Autodesk Inventor part; units mm, degrees
ref_plane "YZ Plane" through (0, 0, 0) normal (1, 0, 0) x (0, 1, 0)
ref_plane "XZ Plane" through (0, 0, 0) normal (0, 1, 0) x (-1, 0, 0)
ref_plane "XY Plane" through (0, 0, 0) normal (0, 0, 1) x (1, 0, 0)
sketch "Sketch1" plane through (0, 0, 0) normal (0, 0, 1) x (1, 0, 0)
  circle A0 centre (0, 0) radius 3.5 construction
  circle A1 centre (0, 0) radius 4.5 construction
  line L0 (0, 0) -> (4.5, 0) construction
  line L1 (4.5, 0) -> (4.5, 3.5) construction
  line L2 (4.5, 3.5) -> (0, 3.5) construction
  line L3 (0, 3.5) -> (0, 0) construction
  line L4 (4.5, 3.5) -> (-4.5, 3.5)
  line L5 (-4.5, 3.5) -> (-4.5, -3.5)
  line L6 (-4.5, -3.5) -> (4.5, -3.5)
  line L7 (4.5, -3.5) -> (4.5, 3.5)
  line L8 (-4.5, 3.5) -> (-6, 3.5) construction
  line L9 (-6, 3.5) -> (-6, -3.5) construction
  line L10 (-6, -3.5) -> (-4.5, -3.5) construction
  line L11 (-4.5, -3.5) -> (-4.5, 3.5) construction
  line L12 (-6, 3.5) -> (4.5, 3.5) construction
  line L13 (4.5, 3.5) -> (4.5, 4.3) construction
  line L14 (4.5, 4.3) -> (-6, 4.3) construction
  line L15 (-6, 4.3) -> (-6, 3.5) construction
  line L16 (-6, -3.5) -> (4.5, -3.5) construction
  line L17 (4.5, -3.5) -> (4.5, -4.3) construction
  line L18 (4.5, -4.3) -> (-6, -4.3) construction
  line L19 (-6, -4.3) -> (-6, -3.5) construction
  line L20 (4.5, -4.3) -> (5.3, -4.3) construction
  line L21 (5.3, -4.3) -> (5.3, 4.3) construction
  line L22 (5.3, 4.3) -> (4.5, 4.3) construction
  line L23 (4.5, 4.3) -> (4.5, -4.3) construction
  line L24 (-6, 4.3) -> (5.3, 4.3)
  line L25 (5.3, 4.3) -> (5.3, -4.3)
  line L26 (5.3, -4.3) -> (-6, -4.3)
  line L27 (-6, -4.3) -> (-6, 4.3)
  dimension "d0" = 7
  dimension "d1" = 9
  dimension "d2" = 4.5
  dimension "d3" = 3.5
  dimension "d4" = 1.5
  dimension "d5" = 0.8
  dimension "d6" = 0.8
  dimension "d7" = 0.8
extrude "Extrusion1" add sketch "Sketch1" along normal blind 3.5
sketch "Sketch2" plane through (0, 0, 3.5) normal (0, 0, 1) x (1, 0, 0)
  line L0 (5.3, -4.3) -> (-6, -4.3)
  line L1 (-6, 4.3) -> (-4.5, 4.3)
  line L2 (-4.5, 4.3) -> (-4.5, -4.3)
  line L3 (-4.5, -4.3) -> (-6, -4.3)
  line L4 (-6, -4.3) -> (-6, 4.3)
  point P0 (0, 0)
extrude "Extrusion2" cut sketch "Sketch2" against normal blind 2.25
sketch "Sketch3" plane through (0, 0, 3.5) normal (0, 0, 1) x (1, 0, 0)
  line L0 (-4.5, -3.5) -> (-4.5, -4.3)
  line L1 (5.3, -4.3) -> (-4.5, -4.3)
  line L2 (5.3, 4.3) -> (5.3, -4.3)
  line L3 (-4.5, 4.3) -> (5.3, 4.3) construction
  line L4 (5.3, 4.3) -> (5.3, 3.9) construction
  line L5 (5.3, 3.9) -> (-4.5, 3.9) construction
  line L6 (-4.5, 3.9) -> (-4.5, 4.3) construction
  line L7 (5.3, 4.3) -> (4.9, 4.3) construction
  line L8 (4.9, 4.3) -> (4.9, -4.3) construction
  line L9 (4.9, -4.3) -> (5.3, -4.3) construction
  line L10 (5.3, -4.3) -> (5.3, 4.3) construction
  line L11 (5.3, -4.3) -> (-4.5, -4.3) construction
  line L12 (-4.5, -4.3) -> (-4.5, -3.9) construction
  line L13 (-4.5, -3.9) -> (5.3, -3.9) construction
  line L14 (5.3, -3.9) -> (5.3, -4.3) construction
  line L15 (-4.5, 3.9) -> (-4.5, 4.3)
  line L16 (5.3, 4.3) -> (5.3, -4.3)
  line L17 (-4.5, -4.3) -> (-4.5, -3.9)
  line L18 (4.9, -3.9) -> (4.9, 3.9)
  line L19 (4.9, 3.9) -> (-4.5, 3.9)
  line L20 (-4.5, 4.3) -> (5.3, 4.3)
  line L21 (4.9, -3.9) -> (-4.5, -3.9)
  line L22 (-4.5, -4.3) -> (5.3, -4.3)
  point P0 (0, 0)
  dimension "d12" = 0.4
  dimension "d13" = 0.4
  dimension "d14" = 0.4
extrude "Extrusion3" cut sketch "Sketch3" against normal blind 0.8
sketch "Sketch4" plane through (-6, -4.3, 0) normal (0, -1, 0) x (1, 0, 0)
  line L0 (11.3, 2.7) -> (1.5, 2.7)
  line L1 (11.3, 0) -> (0, 0)
  line L2 (12.285, 1.4959) -> (-1.3636, 1.4959) construction
  line L3 (6, 1.4959) -> (8, 1.4959) construction
  line L4 (8, 2.7) -> (6, 2.7) construction
  line L5 (8, 2.7) -> (4, 2.7)
  line L6 (1.5, 2.7) -> (2.5, 2.7) construction
  line L7 (2.5, 2.7) -> (2.5, 0) construction
  line L8 (2.5, 0) -> (1.5, 0) construction
  line L9 (1.5, 0) -> (1.5, 2.7) construction
  line L10 (2.5, 2.7) -> (6.5, 2.7)
  line L11 (6.5, 2.7) -> (6.5, 0)
  line L12 (6.5, 0) -> (2.5, 0)
  line L13 (2.5, 0) -> (2.5, 2.7)
  point P0 (6, 0)
  point P1 (4, 0)
  dimension "d29" = 1
  dimension "d30" = 4
extrude "Extrusion4" add sketch "Sketch4" along normal blind 4
fillet "Fillet1" radius 1 14 edges at (5.3, -4.3, 1.35) (4.9, -3.9, 3.1) (-6, -4.3, 0.625) (-6, 4.3, 0.625) (4.9, 3.9, 3.1) (5.3, 4.3, 1.35) (-3.5, -4.3, 1.35) (0.5, -4.3, 1.35) (0.5, -8.3, 1.35) (-3.5, -8.3, 1.35) (4.5, 3.5, 1.75) (4.5, -3.5, 1.75) (-4.5, 3.5, 0.625) (-4.5, -3.5, 0.625)
sketch "Sketch6" plane through (0, 0, 2.7) normal (0, 0, 1) x (1, 0, 0)
  point P0 (0, 0)
  point P1 (-1.5, -6.3)
hole "Hole2" at (-1.5, -6.3, 2.7) direction (0, 0, -1) diameter 1.1938 end through all
sketch "Sketch7" plane through (-4.5, 3.5, 1.25) normal (-1, 0, 0) x (0, 0, 1)
  line L0 (0, 0) -> (2.25, 0)
  line L1 (2.25, 0.4) -> (1.45, 0.4)
  line L2 (1.45, 0.4) -> (1.45, 0)
  line L3 (1.45, 0) -> (2.25, 0)
  line L4 (2.25, 0) -> (2.25, 0.4)
  point P0 (-1.25, -3.5)
extrude "Extrusion5" cut sketch "Sketch7" against normal blind 1
sketch "Sketch8" plane through (-4.5, -3.5, 1.25) normal (-1, 0, 0) x (0, 0, 1)
  line L0 (2.25, 0) -> (1.45, 0)
  line L1 (1.45, 0) -> (1.45, -0.4)
  line L2 (1.45, -0.4) -> (2.25, -0.4)
  line L3 (2.25, -0.4) -> (2.25, 0)
  point P0 (-1.25, 3.5)
extrude "Extrusion6" cut sketch "Sketch8" against normal blind 1
properties part number "window_f"
Geometry check sheet. Reference: the model listing, model coordinates, mm. A direction names the side the tool comes from. Give positions to 0.01 mm unless a question says otherwise; leave off trailing zeros. Loops run counter-clockwise (first coordinate to the right, second up) from the corner with the lowest first, then second, coordinate; pieces in that order, holes last. Notation, with made-up numbers: M -8.75,46 L 2.25,46 A13 ccw 2.25,66 Z; hole C -19.5,-10 d1. An arc over 180 degrees is marked long. Answer as CSV lines item,"result".
Item 1: Cross-section at B-B on z = 2.25. Record the cut outline in (x, y).
Values:
outline,"M -4.5,-4.3 A1 cw -3.5,-5.3 L -3.5,-7.3 A1 ccw -2.5,-8.3 L -0.5,-8.3 A1 ccw 0.5,-7.3 L 0.5,-5.3 A1 cw 1.5,-4.3 L 4.3,-4.3 A1 ccw 5.3,-3.3 L 5.3,3.3 A1 ccw 4.3,4.3 L -4.5,4.3 L -4.5,3.5 L 3.5,3.5 A1 cw 4.5,2.5 L 4.5,-2.5 A1 cw 3.5,-3.5 L -4.5,-3.5 Z; hole C -1.5,-6.3 d1.19"
Item 2: Cross-section at A-A on x = -1.5. Record the cut outline in (y, z).
Values:
outline,"M -8.3,0 L -6.9,0 L -6.9,2.7 L -8.3,2.7 Z; M -5.7,0 L -3.5,0 L -3.5,3.5 L -3.9,3.5 L -3.9,2.7 L -5.7,2.7 Z; M 3.5,0 L 4.3,0 L 4.3,2.7 L 3.9,2.7 L 3.9,3.5 L 3.5,3.5 Z"
Item 3: Cross-section at C-C on y = -6.3. Record the cut outline in (x, z).
Values:
outline,"M -3.5,0 L -2.1,0 L -2.1,2.7 L -3.5,2.7 Z; M -0.9,0 L 0.5,0 L 0.5,2.7 L -0.9,2.7 Z"
Item 4: Material ranges on line 1 (Y direction, x = -1.5, z = 1.3); line 2 (X direction, y = -6.3, z = 0.95); line 3 (Y direction, x = -2, z = 0.75), recorded low to high.
Values:
line 1,"y = -8.3 to -6.9, -5.7 to -3.5, 3.5 to 4.3"
line 2,"x = -3.5 to -2.1, -0.9 to 0.5"
line 3,"y = -8.3 to -6.63, -5.97 to -3.5, 3.5 to 4.3"
Item 5: Release check for a two-part mould opening along Y. For faces 1 (the cylindrical face through (4.215, 3.199, 1.774)), 2 (the flat face through (0, 4.3, 1)), 3 (the cylindrical face through (-3.215, -7.999, 1.369)) record: pulls with the +Y half, pulls with the -Y half, needs draft (parallel to the pull), parting line crosses it, or undercut.
Values:
face 1,"undercut"
face 2,"pulls with the +Y half"
face 3,"pulls with the -Y half"
Item 6: Cross-section at D-D on x = 0.25. Record the cut outline in (y, z), and give its area (3 significant figures).
Values:
outline,"M -7.96,0 L -3.5,0 L -3.5,3.5 L -3.9,3.5 L -3.9,2.7 L -7.96,2.7 Z; M 3.5,0 L 4.3,0 L 4.3,2.7 L 3.9,2.7 L 3.9,3.5 L 3.5,3.5 Z"
area,"14.8 mm²"
Item 7: Depth check by flat-ended pin: P1, Ø1, axis at x = -1, y = -5.5, coming from the +Z side; P2, Ø2, axis at y = -6.5, z = 2, coming from the -X side; P3, Ø2, axis at x = 3.5, z = 1, coming from the -Y side. Enter the tip coordinate at first touch or a pass-through.
Values:
P1,"stops at z = 2.7"
P2,"stops at x = -3.5"
P3,"stops at y = -4.3"
Item 8: Access from +Z, -Z, +X, -X, +Y, -Y to the whole of each face (thin tool, end or side, straight path). Record for faces 4 (the flat face through (-3.5, -6, 1)), 5 (the cylindrical face through (4.199, -3.215, 1.774)), 6 (the cylindrical face through (4.615, -3.599, 3.094)).
Values:
face 4,"+Z, -Z, -X, -Y"
face 5,"+Z, -Z"
face 6,"+Z, +X, -Y"
